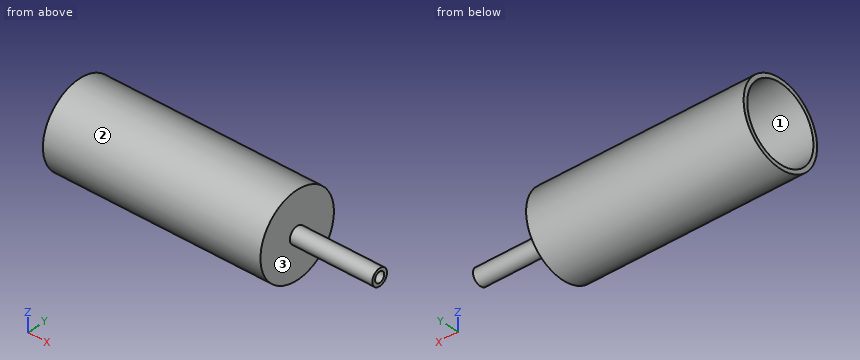
```python
from build123d import *
from build123d.topology import SkipClean

# Parameters (mm, degrees)
CUT_EXTRUDE1_START  = -0.5
CUT_EXTRUDE1_DEPTH  = 2
CIRPATTERN1_COUNT   = 8
SKETCH3_R           = 0.75
SKETCH3_R_2         = 0.625
BOSS_EXTRUDE1_DEPTH = 2.5
CUT_EXTRUDE2_START  = -2.5
SKETCH4_R           = 0.625
CUT_EXTRUDE2_DEPTH  = 2.5
BOSS_EXTRUDE2_START = 10
SKETCH5_R           = 1
SKETCH5_R_2         = 0.625
BOSS_EXTRUDE2_DEPTH = 10


with BuildPart() as part:
    # Sketch1 → Revolve1 (revolve)
    with BuildSketch(Plane.XY):
        Polygon((0, 0), (0, 1), (-1, 2), (-7, 2), (-7, 4), (-10, 4), (-10, 3), (-13, 3), (-14.5, 4.5), (-24.88, 4.5), (-24.88, 5), (1.5, 5), (1.5, 0), align=None)
    revolve(axis=Axis((1.5, 0, 0), (-1, 0, 0)))

    # Sketch2 → Cut-Extrude1 (cut)
    with BuildSketch(Plane.ZY.offset(7).offset(CUT_EXTRUDE1_START)):
        with BuildLine():
            Line((-2, -0.1), (-3.9, -0.1))
            ThreePointArc((-3.9, -0.1), (-4, 0), (-3.9, 0.1))
            Line((-3.9, 0.1), (-2, 0.1))
            ThreePointArc((-2, 0.1), (-1.9, 0), (-2, -0.1))
        make_face()
    cut_extrude1 = extrude(amount=CUT_EXTRUDE1_DEPTH, mode=Mode.SUBTRACT)

    # CirPattern1: Cut-Extrude1 ×8 about axis
    cirpattern1_axis = Axis((0, 0, 0), (1, 0, 0))
    for i in range(1, CIRPATTERN1_COUNT):
        add(cut_extrude1.rotate(cirpattern1_axis, i * 360 / CIRPATTERN1_COUNT), mode=Mode.SUBTRACT)

    # Sketch3 → Boss-Extrude1 (add)
    with BuildSketch(Plane.ZY):
        with Locations(Location((0, 0, 0), (0, 0, 270))):
            Circle(SKETCH3_R)
        with Locations(Location((0, 0, 0), (0, 0, 270))):
            Circle(SKETCH3_R_2, mode=Mode.SUBTRACT)
    extrude(amount=BOSS_EXTRUDE1_DEPTH)

    # Sketch4 → Cut-Extrude2 (cut)
    with BuildSketch(Plane.ZY.offset(CUT_EXTRUDE2_START)):
        with Locations(Location((0, 0, 0), (0, 0, 90))):
            Circle(SKETCH4_R)
    extrude(amount=CUT_EXTRUDE2_DEPTH, mode=Mode.SUBTRACT)

    # Sketch5 → Boss-Extrude2 (add)
    with SkipClean():  # the faces are left unmerged after this step: merging them gives an invalid solid
        with BuildSketch(Plane(origin=(1.5, 0, 0), x_dir=(0, 0, -1), z_dir=(1, 0, 0)).offset(BOSS_EXTRUDE2_START)):
            with Locations(Location((0, 0, 0), (0, 0, 90))):
                Circle(SKETCH5_R)
            with Locations(Location((0, 0, 0), (0, 0, 90))):
                Circle(SKETCH5_R_2, mode=Mode.SUBTRACT)
        extrude(amount=-BOSS_EXTRUDE2_DEPTH)


solid = part.part
```
The listing builds one solid part. Answer for the finished solid, in the listing's coordinates (mm). Face numbers are marked on the shaded views. Round coordinates to 2 decimals unless told otherwise and drop trailing zeros. Write each loop counter-clockwise with the first axis right and the second up, starting at its lowest first coordinate (ties: lowest second). Pieces come first, ordered by that corner, then holes. Notation, with made-up numbers: (76, -2.5) -> (94, -2.5) arc R27 cw to (94, 25.5) -> close; hole circle Ø9 at (89, -4). An arc over 180 degrees is marked (long way). Write item = value, one per line.
1) Section A-A on x = 4.5 is taken. Write down the section's boundary in (y, z) (3 decimals), plus the area to 3 significant figures.
Check values:
outline = circle Ø2 at (0, 0); hole circle Ø1.25 at (0, 0)
area = 1.91 mm²
2) Section B-B on x = -22 is taken. Write down the section's boundary in (y, z).
Check values:
outline = circle Ø10 at (0, 0); hole circle Ø9 at (0, 0)
3) Straight lines are drawn through the part: line 1 along Z through (x, y) = (-10.6, 0); line 2 along Z through (x, y) = (-9.4, 0); line 3 along Y through (x, z) = (-5.7, 0). For each, find the intervals that lie inside material, in ascending order. Write a range as [from, to].
Check values:
line_1 = [-5, -3], [3, 5]
line_2 = [-5, -4], [4, 5]
line_3 = [-5, -2], [2, 5]
4) Given pin 1 (0.6 mm diameter, centred on y = -0.5, z = -0.5, fed in from -X); pin 2 (2 mm diameter, centred on x = -21, y = 2, fed in from -Z); pin 3 (0.8 mm diameter, centred on y = 2, z = -2, fed in from -X); pin 4 (1.1 mm diameter, centred on y = 0, z = 0, fed in from +X), each flat-ended and moving along its own axis, determine where each tip first touches the part or whether it passes through.
Check values:
pin_1 = -2.5
pin_2 = -4.9
pin_3 = -13.23
pin_4 = through
5) For a pull along Y with two mould halves and no side action, classify the marked faces 1, 2 and 3 as released by +Y, released by -Y, zero draft, split by the parting line, or undercut.
Check values:
face_1 = undercut
face_2 = split by the parting line
face_3 = zero draft
